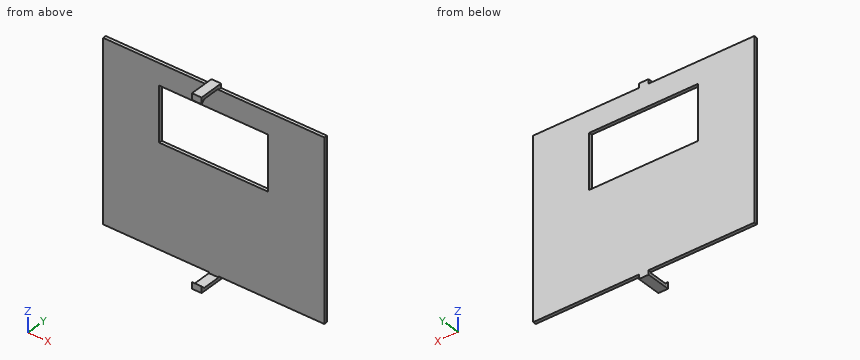
from build123d import *

# Parameters (mm, degrees)
SKETCH1_W           = 103
SKETCH1_H           = 83
BOSS_EXTRUDE1_DEPTH = 1.5
BOSS_EXTRUDE2_DEPTH = 2.25
SKETCH3_W           = 50.8
SKETCH3_H           = 25.4
CUT_EXTRUDE1_DEPTH  = 1.5


with BuildPart() as part:
    # Sketch1 → Boss-Extrude1 (new body)
    with BuildSketch(Plane(origin=(0, 0, 0), x_dir=(1, 0, 0), z_dir=(0, 1, 0))):
        with Locations((18.292349727, -12.091530055)):
            Rectangle(SKETCH1_W, SKETCH1_H)
    extrude(amount=BOSS_EXTRUDE1_DEPTH)

    # Sketch2 → Boss-Extrude2 (add, symmetric)
    with BuildSketch(Plane(origin=(18.292349727, 0, 0), x_dir=(0, 0, -1), z_dir=(1, 0, 0))):
        Polygon((-53.591530055, 1.5), (-55.591530055, 1.5), (-55.591530055, -10), (-52.592463679, -10), (-54.091530055, -8.500933624), (-54.091530055, 0), (-53.591530055, 0), align=None)
        Polygon((29.408469945, 0), (29.408469945, 1.5), (31.408469945, 1.5), (31.408469945, -10), (28.409403569, -10), (29.908469945, -8.500933624), (29.908469945, 0), align=None)
    extrude(amount=BOSS_EXTRUDE2_DEPTH, both=True)

    # Sketch3 → Cut-Extrude1 (cut)
    with BuildSketch(Plane(origin=(0, 1.5, 0), x_dir=(1, 0, 0), z_dir=(0, 1, 0))):
        with Locations((18.292349727, -30.891530055)):
            Rectangle(SKETCH3_W, SKETCH3_H)
    extrude(amount=-CUT_EXTRUDE1_DEPTH, mode=Mode.SUBTRACT)


solid = part.part
Verification items for the finished model (mm, model axes). Round coordinates to 2 decimals unless told otherwise and drop trailing zeros. Order: outer loops, then holes, each group sorted by start corner. A loop starts at its lowest first (then second) coordinate and runs counter-clockwise, first axis right, second up.
1. Section check B-B on y = -5. Record the cut outline in (x, z), then the cut area to 3 significant figures.
Final values:
outline: (16.04, -31.41) - (20.54, -31.41) - (20.54, -29.91) - (16.04, -29.91) - close; (16.04, 54.09) - (20.54, 54.09) - (20.54, 55.59) - (16.04, 55.59) - close
area: 13.5 mm2
2. Thickness scan on L1, parallel to Z at x = 19, y = -7.5; L2, parallel to Y at x = 33, z = -17; L3, parallel to Z at x = 64.5, y = 0.5. Record the ranges inside material, lowest first.
Final values:
L1: z = -31.41 to -29.91, 54.09 to 55.59
L2: y = 0 to 1.5
L3: z = -29.41 to 53.59
3. Go/stop test with flat-tipped pins: P1, Ø1.5, axis at y = -6, z = -29.5, coming from the -X side; P2, Ø2, axis at x = -6.5, z = 13, coming from the -Y side; P3, Ø0.8, axis at x = 36, y = 0.5, coming from the -Z side; P4, Ø6, axis at y = -1.5, z = 8.5, coming from the +X side. Record where each tip stops, or that it passes through.
Final values:
P1: stops at x = 16.04
P2: stops at y = 0
P3: stops at z = -29.41
P4: stops at x = 69.79
4. Section check D-D on z = -13. Record the cut outline in (x, y), then the cut area to 4 significant figures.
Final values:
outline: (-33.21, 0) - (69.79, 0) - (69.79, 1.5) - (-33.21, 1.5) - close
area: 154.5 mm2
5. Section check C-C on x = 57. Record the cut outline in (y, z), then the cut area to 4 significant figures.
Final values:
outline: (0, -29.41) - (1.5, -29.41) - (1.5, 53.59) - (0, 53.59) - close
area: 124.5 mm2
6. Section check A-A on z = 39. Record the cut outline in (x, y).
Final values:
outline: (-33.21, 0) - (-7.11, 0) - (-7.11, 1.5) - (-33.21, 1.5) - close; (43.69, 0) - (69.79, 0) - (69.79, 1.5) - (43.69, 1.5) - close
